The model under review builds one solid part; all positions refer to its coordinate system, in mm. A direction names the side the tool comes from. Give positions to 0.01 mm unless a question says otherwise; leave off trailing zeros. Order: outer loops, then holes, each group sorted by start corner. A loop starts at its lowest first (then second) coordinate and runs counter-clockwise, first axis right, second up. Notation, with made-up numbers: (-27, 6.5) - (15, 6.5) arc R24 cw to (15, 40.5) - close; hole circle Ø4 at (65, 9.25). An arc over 180 degrees is marked (long way). Put each result on its own line as item: value.
```python
from build123d import *

# Parameters (mm, degrees)
F4_DEPTH      = 30
F4_DEPTH_BACK = -2
F5_W          = 100
F5_H          = 100
F6_DEPTH      = 2


with BuildPart() as f2:
    # F0 (on Front) → F2 (revolve)
    with BuildSketch(Plane.XZ):
        Polygon((0, 2), (0, 0), (19.877748, 0), (36.150404, 29), (34.150404, 29), (19, 2), align=None)
    revolve(axis=Axis((0, 0, 10.899935), (0, 0, 1)))

    # F3 (on Top) → F4 (cut, two sides)
    with BuildSketch(Plane.XY) as f4_sk:
        Polygon((-72.002242, 5), (-72.002242, 0), (-72.002242, -5), (-5, -5), (-5, -72.002242), (0, -72.002242), (5, -72.002242), (5, -5), (72.002242, -5), (72.002242, 0), (72.002242, 5), (5, 5), (5, 72.002242), (0, 72.002242), (-5, 72.002242), (-5, 5), align=None)
    extrude(amount=F4_DEPTH, mode=Mode.SUBTRACT)
    extrude(f4_sk.sketch, amount=-F4_DEPTH_BACK, mode=Mode.SUBTRACT)

    # F5 (on Top) → F6 (join)
    with BuildSketch(Plane.XY):
        Rectangle(F5_W, F5_H)
    extrude(amount=F6_DEPTH)


solid = f2.part
```
(1) Wall thickness on L1, parallel to Z at x = 5.5, y = 4.5; L2, parallel to Y at x = 22.5, z = 19.5; L3, parallel to X at y = 24, z = 21.5: over which ranges is each line inside the solid? List them lowest first.
The answers:
L1: 0 to 2
L2: -21.06 to -18.01, 18.01 to 21.06
L3: -21.08 to -17.9, 17.9 to 21.08
(2) For faces 1 (the flat face through (5, -27, 15)), 2 (the flat face through (-1, 1, 2)), 3 (the conical face through (-18.88, -18.55, 15.31)), list the 3-axis set-ups (+Z, -Z, +X, -X, +Y, -Y) from which the entire face can be reached by the end or side of a thin tool; tool diameter is ignored.
The answers:
face 1: +Z, +Y, -Y
face 2: none
face 3: +Z
(3) Clearance check with flat-ended pins moving along their axes: pin 1 Ø5 at (y, z) = (-25, 21.5) entering from +X; pin 2 Ø6 at (x, z) = (-4, 10) entering from -Y; pin 3 Ø14 at (y, z) = (-30.5, 16) entering from -X. State where each tip first meets the part, or that it passes through.
The answers:
pin 1: x = 23.36
pin 2: y = -26.61
pin 3: x = -18.83
(4) Take a section at C-C, the plane z = 24.75. Write out the cut boundary in (x, y), then the cut area to 3 significant figures.
The answers:
outline: (-33.39, -5) arc R33.77 ccw to (-5, -33.39) - (-5, -31.37) arc R31.77 cw to (-31.37, -5) - close; (-33.39, 5) - (-31.37, 5) arc R31.77 cw to (-5, 31.37) - (-5, 33.39) arc R33.77 ccw to start; (5, -33.39) arc R33.77 ccw to (33.39, -5) - (31.37, -5) arc R31.77 cw to (5, -31.37) - close; (5, 31.37) arc R31.77 cw to (31.37, 5) - (33.39, 5) arc R33.77 ccw to (5, 33.39) - close
area: 331 mm^2
(5) The part is to be moulded in two halves that separate along Y. For faces 4 (the conical face through (18.88, 18.55, 15.31)), 5 (the conical face through (-18.55, 18.88, 15.31)), 6 (the flat face through (-5, 27, 15)), say which applies: pulls with the +Y half, pulls with the -Y half, needs draft (parallel to the pull), parting line crosses it, or undercut.
The answers:
face 4: undercut
face 5: undercut
face 6: needs draft
(6) Take a section at A-A, the plane z = 14.5. Write out the cut boundary in (x, y).
The answers:
outline: (-27.56, -5) arc R28.01 ccw to (-5, -27.56) - (-5, -25.53) arc R26.01 cw to (-25.53, -5) - close; (-27.56, 5) - (-25.53, 5) arc R26.01 cw to (-5, 25.53) - (-5, 27.56) arc R28.01 ccw to start; (5, -27.56) arc R28.01 ccw to (27.56, -5) - (25.53, -5) arc R26.01 cw to (5, -25.53) - close; (5, 25.53) arc R26.01 cw to (25.53, 5) - (27.56, 5) arc R28.01 ccw to (5, 27.56) - close
(7) Take a section at D-D, the plane x = -39. Write out the cut boundary in (y, z).
The answers:
outline: (-50, 0) - (50, 0) - (50, 2) - (-50, 2) - close
(8) Take a section at B-B, the plane x = 30. Count the separate pieces of the cut face and the enclosed holes in it, then the cut area to 3 significant figures.
The answers:
separate pieces: 3
enclosed holes: 0
area: 295 mm^2
